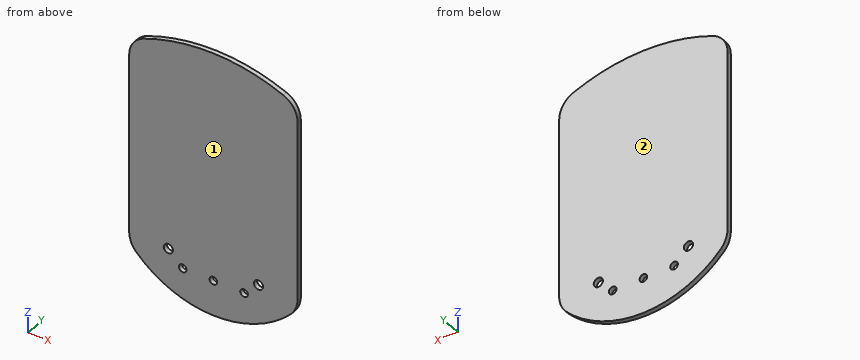
from build123d import *

# Parameters (mm, degrees)
SKETCH2_R           = 3
SKETCH2_R_2         = 2.5
BOSS_EXTRUDE1_DEPTH = 3


with BuildPart() as part:
    # Sketch2 → Boss-Extrude1 (new body)
    with BuildSketch(Plane(origin=(0, 0, 0), x_dir=(1, 0, 0), z_dir=(0, 1, 0))):
        with BuildLine():
            Line((-54.843939578, -82.950592443), (-54.843939578, 33.080710792))
            ThreePointArc((-54.843939578, 33.080710792), (-53.629479142, 38.690320935), (-50.582114931, 43.554086088))
            ThreePointArc((-50.582114931, 43.554086088), (0, 64.876726435), (50.582114931, 43.554086088))
            ThreePointArc((50.582114931, 43.554086088), (53.581553542, 38.670819055), (54.843939578, 33.080710792))
            Line((54.843939578, 33.080710792), (54.843939578, -82.950592443))
            ThreePointArc((54.843939578, -82.950592443), (52.270146994, -91.352340431), (45.432023677, -96.870840864))
            ThreePointArc((45.432023677, -96.870840864), (0, -105.649395093), (-45.432023677, -96.870840864))
            ThreePointArc((-45.432023677, -96.870840864), (-52.270146994, -91.352340431), (-54.843939578, -82.950592443))
        make_face()
        with Locations((29.359626422, 33.197024949)):
            Circle(SKETCH2_R, mode=Mode.SUBTRACT)
        with Locations((-29.359626422, 33.197024949)):
            Circle(SKETCH2_R, mode=Mode.SUBTRACT)
        with Locations((0, 42.202367755)):
            Circle(SKETCH2_R_2, mode=Mode.SUBTRACT)
        with Locations((20, 42.202367755)):
            Circle(SKETCH2_R_2, mode=Mode.SUBTRACT)
        with Locations((-20, 42.202367755)):
            Circle(SKETCH2_R_2, mode=Mode.SUBTRACT)
    extrude(amount=BOSS_EXTRUDE1_DEPTH)


solid = part.part
Check sheet for the modelled part. Datum: model origin and axes. Units: mm. Face numbers are marked on the shaded views. Round coordinates to 2 decimals unless told otherwise and drop trailing zeros. Order: outer loops, then holes, each group sorted by start corner. A loop starts at its lowest first (then second) coordinate and runs counter-clockwise, first axis right, second up.
(1) Go/stop test with a flat-tipped pin: P1, Ø1.5, axis at x = 38.5, y = 1, coming from the -Z side. Record where the tip stops, or that it passes through.
(2) Cross-section at A-A, the plane x = 0. Enter the section's corners in (y, z).
(3) Scan lines: probe 1 along Z at (x, y) = (-20, 1.8); probe 2 along Z at (x, y) = (27.5, 0.7); probe 3 along Z at (x, y) = (-3, 2.1). Record each from-to range of solid material in increasing order.
(4) Cross-section at C-C, the plane x = 20. Enter the section's corners in (y, z), and give its area (3 significant figures).
(5) Cross-section at D-D, the plane x = 34. Enter the section's corners in (y, z).
(6) Cross-section at B-B, the plane y = 0.7. Enter the section's corners in (x, z).
(7) Draft check along Y on the marked faces 1 and 2. Enter one of: pulls with the +Y half, pulls with the -Y half, needs draft (parallel to the pull), parting line crosses it, or undercut.
Check sheet entries:
1. P1: stops at z = -53.95
2. outline: (0, -64.88) - (3, -64.88) - (3, -44.7) - (0, -44.7) - close; (0, -39.7) - (3, -39.7) - (3, 105.65) - (0, 105.65) - close
3. probe 1: z = -61.99 to -44.7, -39.7 to 104
3. probe 2: z = -59.31 to -35.55, -30.84 to 102.51
3. probe 3: z = -64.81 to 105.61
4. outline: (0, -61.99) - (3, -61.99) - (3, -44.7) - (0, -44.7) - close; (0, -39.7) - (3, -39.7) - (3, 104) - (0, 104) - close
4. area: 483 mm2
5. outline: (0, -56.16) - (3, -56.16) - (3, 100.81) - (0, 100.81) - close
6. outline: (-54.84, -33.08) arc R16.65 ccw to (-50.58, -43.55) arc R70.66 ccw to (50.58, -43.55) arc R17.51 ccw to (54.84, -33.08) - (54.84, 82.95) arc R15 ccw to (45.43, 96.87) arc R121.95 ccw to (-45.43, 96.87) arc R15 ccw to (-54.84, 82.95) - close; hole circle Ø6 at (-29.36, -33.2); hole circle Ø5 at (-20, -42.2); hole circle Ø5 at (0, -42.2); hole circle Ø5 at (20, -42.2); hole circle Ø6 at (29.36, -33.2)
7. face 1: pulls with the -Y half
7. face 2: pulls with the +Y half
